from build123d import *

# Parameters (mm, degrees)
SKETCH101_R           = 14
SKETCH101_R_2         = 6.5
PAD060_DEPTH          = 11
SKETCH102_R           = 7.15
POCKET039_DEPTH       = 4
SKETCH103_R           = 1.75
POCKET040_DEPTH       = 93.19589
POLARPATTERN021_COUNT = 6
SKETCH104_R           = 2.05
POCKET041_DEPTH       = 7
POLARPATTERN022_COUNT = 3
CHAMFER037_SIZE       = 0.25
CHAMFER036_SIZE       = 0.4


with BuildPart() as part:
    # Sketch101 → Pad060 (new body)
    with BuildSketch(Plane.XY):
        Circle(SKETCH101_R)
        Circle(SKETCH101_R_2, mode=Mode.SUBTRACT)
    extrude(amount=PAD060_DEPTH)

    # Sketch102 → Pocket039 (cut)
    with BuildSketch(Plane.XY):
        Circle(SKETCH102_R)
    extrude(amount=POCKET039_DEPTH, mode=Mode.SUBTRACT)

    # Sketch103 → Pocket040 (cut, through all)
    with BuildSketch(Plane.XY):
        with Locations((0, 10.5)):
            Circle(SKETCH103_R)
    pocket040 = extrude(amount=POCKET040_DEPTH, mode=Mode.SUBTRACT)

    # PolarPattern021: Pocket040 ×6 about axis
    polarpattern021_axis = Axis((0, 0, 0), (0, 0, 1))
    for i in range(1, POLARPATTERN021_COUNT):
        add(pocket040.rotate(polarpattern021_axis, i * 360 / POLARPATTERN021_COUNT), mode=Mode.SUBTRACT)

    # Sketch104 (on Plane of DatumPlane006) → Pocket041 (cut)
    with BuildSketch(Plane.XY.offset(11)):
        with Locations((0, -10.5)):
            Circle(SKETCH104_R)
    pocket041 = extrude(amount=-POCKET041_DEPTH, mode=Mode.SUBTRACT)

    # PolarPattern022: Pocket041 ×3 about axis
    polarpattern022_axis = Axis((0, 0, 11), (0, 0, 1))
    for i in range(1, POLARPATTERN022_COUNT):
        add(pocket041.rotate(polarpattern022_axis, i * 360 / POLARPATTERN022_COUNT), mode=Mode.SUBTRACT)

    # Chamfer037
    chamfer037_edges = [part.edges().sort_by_distance(p)[0] for p in [
        (1.75, -10.5, 4),
        (8.218267, 6.765544, 4),
        (-9.968267, 3.734456, 4),
    ]]
    chamfer(chamfer037_edges, length=CHAMFER037_SIZE)

    # Chamfer036
    chamfer036_edges = [part.edges().sort_by_distance(p)[0] for p in [
        (-14, 0, 11),
        (-8.218267, -6.765544, 11),
        (-2.05, -10.5, 11),
        (9.968267, -3.734456, 11),
        (-8.068267, 7.025352, 11),
        (-6.5, 0, 11),
        (10.118267, 3.474648, 11),
        (-1.75, 10.5, 11),
        (-14, 0, 0),
        (1.75, -10.5, 0),
        (-8.218267, -6.765544, 0),
        (-7.15, 0, 0),
        (9.968267, -3.734456, 0),
        (-9.968267, 3.734456, 0),
        (-1.75, 10.5, 0),
        (8.218267, 6.765544, 0),
    ]]
    chamfer(chamfer036_edges, length=CHAMFER036_SIZE)


solid = part.part
Model file for the job. Use its own axes, mm. A direction names the side the tool comes from. Give positions to 0.01 mm unless a question says otherwise; leave off trailing zeros. Order: outer loops, then holes, each group sorted by start corner. A loop starts at its lowest first (then second) coordinate and runs counter-clockwise, first axis right, second up. Notation, with made-up numbers: (-3.5, 2.25) - (48.5, 2.25) arc R23 cw to (48.5, 29.25) - close; hole circle Ø4 at (44, 71.5). An arc over 180 degrees is marked (long way). Write item = value, one per line. Start each with the question number.
1. Probe line 1 along Y through (x, z) = (-1, 4.75); line 2 along Y through (x, z) = (8, 4.25); line 3 along Y through (x, z) = (0.5, 4.75). List the from-to ranges inside material, lowest first.
2. Cut at C-C, the plane x = 10.5. State how many separate pieces and enclosed holes the cut face has, and give its area (3 significant figures).
3. Cut at A-A, the plane y = 0. List the corners of the cut face in (x, z), and give its area (3 significant figures).
4. Drop flat-ended pins along their axis: P1, Ø2, axis at x = -8, z = 3.5, coming from the +Y side; P2, Ø5, axis at x = 3.5, y = -3.5, coming from the -Z side; P3, Ø3, axis at y = 8.5, z = 8, coming from the -X side. Give the stop position or say it passes through.
5. Cut at B-B, the plane z = 7.5. List the corners of the cut face in (x, y), and give its area (3 significant figures).
6. Two-plate mould, pull along Y, no slides. Class faces 3 (the flat face through (3, -6, 4)), 4 (the cylindrical face through (12.932, -5.362, 5.429)): pulls with the +Y half, pulls with the -Y half, needs draft (parallel to the pull), parting line crosses it, or undercut.
7. Which spindle directions (+Z, -Z, +X, -X, +Y, -Y) get a long thin tool onto all of the face, cutting with end or side? Do faces 1 (the cylindrical face through (11, 6, 7)), 2 (the cylindrical face through (-10.482, -6.315, 5.429)). Say none if no direction does.
Taken from the geometry:
q1.line_1 = -13.96 to -12.29, -8.71 to -6.42, 6.42 to 9.06, 11.94 to 13.96
q1.line_2 = -11.49 to -6.62, -3.88 to 3.52, 6.98 to 11.49
q1.line_3 = -13.99 to -12.49, -8.51 to -6.48, 6.48 to 8.82, 12.18 to 13.99
q2.separate_pieces = 3
q2.enclosed_holes = 0
q2.area = 150 mm²
q3.outline = (-14, 0.4) - (-13.6, 0) - (-7.55, 0) - (-7.15, 0.4) - (-7.15, 4) - (-6.5, 4) - (-6.5, 10.6) - (-6.9, 11) - (-13.6, 11) - (-14, 10.6) - close; (6.5, 4) - (7.15, 4) - (7.15, 0.4) - (7.55, 0) - (13.6, 0) - (14, 0.4) - (14, 10.6) - (13.6, 11) - (6.9, 11) - (6.5, 10.6) - close
q3.area = 159 mm²
q4.P1 = 12.12
q4.P2 = 0.1
q4.P3 = -12.12
q5.outline = circle Ø28 at (0, 0); hole circle Ø4.1 at (-9.09, 5.25); hole circle Ø3.5 at (-9.09, -5.25); hole circle Ø13 at (0, 0); hole circle Ø4.1 at (0, -10.5); hole circle Ø3.5 at (0, 10.5); hole circle Ø4.1 at (9.09, 5.25); hole circle Ø3.5 at (9.09, -5.25)
q5.area = 415 mm²
q6.face_3 = undercut
q6.face_4 = parting line crosses it
q7.face_1 = +Z
q7.face_2 = +Z, -Z
